Can you work these out from the model? Positions are in its coordinate system, mm. A direction names the side the tool comes from. Give positions to 0.01 mm unless a question says otherwise; leave off trailing zeros. Write each loop counter-clockwise with the first axis right and the second up, starting at its lowest first coordinate (ties: lowest second). Pieces come first, ordered by that corner, then holes.
1. I'm going to push flat-ended pins straight in: pin 1 (3 mm diameter, centred on x = -2.5, y = 1.5, fed in from +Z); pin 2 (1.5 mm diameter, centred on x = -2.5, y = 1, fed in from -Z); pin 3 (2 mm diameter, centred on x = -1.5, y = 5, fed in from -Z). Where does each tip first touch, or does it pass through?
2. Thinking about a two-plate mould opening in X: for faces 1 (the flat face through (-1.24, 6.35, -1.24)), 2 (the cylindrical face through (0.69, 1.57, 3.1)), 3 (the cylindrical face through (1.38, 3.14, 6.2)), which applies, pulls with the +X half, pulls with the -X half, needs draft (parallel to the pull), parting line crosses it, or undercut?
3. Suppose I cut it at C-C (y = 2.25). Please give me the cut outline in (x, z) (3 decimals).
4. On a 3-axis mill with a long thin cutter (end or side, diameter ignored), from which of +Z, -Z, +X, -X, +Y, -Y can I reach the whole of each face in a straight line? I mean faces 4 (the cylindrical face through (0.34, 4.74, 1.55)), 5 (the flat face through (-1.4, 3.175, -1.4)). Say none if no direction works.
5. If I drill on probe 1 along Z at (x, y) = (0, 1.5) (3 decimals); probe 2 along Z at (x, y) = (0, 4.45); probe 3 along X at (y, z) = (2.25, -1.25), over which ranges is the centre line in solid material (lowest first)?
Autodesk Inventor part; units mm, degrees
ref_plane "YZ Plane" through (0, 0, 0) normal (1, 0, 0) x (0, 1, 0)
ref_plane "XZ Plane" through (0, 0, 0) normal (0, 1, 0) x (-1, 0, 0)
ref_plane "XY Plane" through (0, 0, 0) normal (0, 0, 1) x (1, 0, 0)
sketch "Sketch1" plane through (0, 0, 0) normal (0, 1, 0) x (-1, 0, 0)
  circle A0 centre (0, 0) radius 6.35
  circle A1 centre (0, 0) radius 1.5875
  circle A2 centre (0, 0) radius 3.175
  dimension "d0" = 12.7
  dimension "d1" = 3.175
  dimension "d4" = 6.35
extrude "Extrusion1" add sketch "Sketch1" along normal blind 6.35 contours A0 | A2
extrude "Extrusion2" cut sketch "Sketch1" along normal blind 3.175 contours A1 | A2
fillet "Fillet1" radius 0.4 2 edges at (6.35, 6.35, 0) (6.35, 0, 0)
properties part number "Bumper"
Checks:
1. pin 1: stops at z = 6.27
1. pin 2: stops at z = -6.1
1. pin 3: stops at z = -6.33
2. face 1: needs draft
2. face 2: undercut
2. face 3: parting line crosses it
3. outline: circle Ø12.7 at (0, 0); hole circle Ø6.35 at (0, 0)
4. face 4: +Y, -Y
4. face 5: -Y
5. probe 1: z = -6.35 to -3.175, 3.175 to 6.35
5. probe 2: z = -6.35 to -1.59, 1.59 to 6.35
5. probe 3: x = -6.23 to -2.92, 2.92 to 6.23
